Geometry check sheet. Reference: the model listing, model coordinates, mm. Face numbers are marked on the shaded views. A direction names the side the tool comes from. Coordinates: 2 decimals unless noted, no trailing zeros. Order: outer loops, then holes, each group sorted by start corner. A loop starts at its lowest first (then second) coordinate and runs counter-clockwise, first axis right, second up. Notation, with made-up numbers: (67.5, 87.25) -> (121.5, 87.25) arc R26 cw to (121.5, 110.25) -> close; hole circle Ø11 at (13, 44). An arc over 180 degrees is marked (long way). Answer in a Markdown table with one row per item. Add a question column.
```python
from build123d import *

# Parameters (mm, degrees)
F0_W      = 67.5
F0_H      = 19.4
F1_DEPTH  = 50
F3_DEPTH  = 17.5
F4_R      = 12
F5_DEPTH  = 1.9
F7_DEPTH  = 1.25
F8_DEPTH  = 11
F9_R      = 7
F11_DEPTH = 8
F12_R     = 5
F14_DEPTH = 1.25


with BuildPart() as f1:
    # F0 (on Top) → F1 (new body)
    with BuildSketch(Plane.XY):
        Rectangle(F0_W, F0_H)
    extrude(amount=F1_DEPTH)

    # F2 (on face) → F3 (cut)
    with BuildSketch(Plane.XZ.offset(9.7)):
        with BuildLine():
            Line((-6.1, 31.5), (-6.1, 30.5))
            Line((-6.1, 30.5), (-29.5, 30.5))
            ThreePointArc((-29.5, 30.5), (-31.62132, 29.62132), (-32.5, 27.5))
            Line((-32.5, 27.5), (-32.5, 1.5))
            Line((-32.5, 1.5), (0, 1.5))
            Line((0, 1.5), (32.5, 1.5))
            Line((32.5, 1.5), (32.5, 27.5))
            ThreePointArc((32.5, 27.5), (31.62132, 29.62132), (29.5, 30.5))
            Line((29.5, 30.5), (6.1, 30.5))
            Line((6.1, 30.5), (6.1, 31.5))
            Line((6.1, 31.5), (5.1, 31.5))
            Line((5.1, 31.5), (0, 31.5))
            Line((0, 31.5), (-5.1, 31.5))
            Line((-5.1, 31.5), (-6.1, 31.5))
        make_face()
    extrude(amount=-F3_DEPTH, mode=Mode.SUBTRACT)

    # F4 (on face) → F5 (cut, through all)
    with BuildSketch(Plane.XZ.offset(-7.8)):
        with Locations((0, 16)):
            Circle(F4_R)
    extrude(amount=-F5_DEPTH, mode=Mode.SUBTRACT)

    # F6 (on face) → F7 (cut, through all)
    with BuildSketch(Plane(origin=(-33.75, 0, 0), x_dir=(0, -1, 0), z_dir=(-1, 0, 0))):
        with BuildLine():
            Line((3.45, 26.5), (0.95, 26.5))
            ThreePointArc((0.95, 26.5), (-1.17132, 25.62132), (-2.05, 23.5))
            Line((-2.05, 23.5), (-2.05, 12.5))
            ThreePointArc((-2.05, 12.5), (-1.17132, 10.37868), (0.95, 9.5))
            Line((0.95, 9.5), (3.45, 9.5))
            ThreePointArc((3.45, 9.5), (5.57132, 10.37868), (6.45, 12.5))
            Line((6.45, 12.5), (6.45, 23.5))
            ThreePointArc((6.45, 23.5), (5.57132, 25.62132), (3.45, 26.5))
        make_face()
    extrude(amount=-F7_DEPTH, mode=Mode.SUBTRACT)

    # F2 (on face) → F8 (cut)
    with BuildSketch(Plane.XZ.offset(9.7)):
        Polygon((-5.1, 50), (-5.1, 31.5), (0, 31.5), (5.1, 31.5), (5.1, 50), (0, 50), align=None)
    extrude(amount=-F8_DEPTH, mode=Mode.SUBTRACT)

    # F9
    f9_edges = [f1.edges().sort_by_distance(p)[0] for p in [
        (32.5, -0.95, 1.5),
        (-33.75, 0, 0),
        (-32.5, -0.95, 1.5),
        (33.75, 0, 0),
    ]]
    fillet(f9_edges, radius=F9_R)

    # F10 (on face) → F11 (join)
    with BuildSketch(Plane.XY.offset(50)):
        Polygon((10, 9.7), (0, 9.7), (-10, 9.7), (-10, 2.7), (0, 2.7), (10, 2.7), align=None)
    extrude(amount=F11_DEPTH)

    # F12
    f12_edges = [f1.edges().sort_by_distance(p)[0] for p in [
        (10, 6.2, 58),
        (-10, 6.2, 58),
    ]]
    fillet(f12_edges, radius=F12_R)

    # F13 (on face) → F14 (cut, through all)
    with BuildSketch(Plane.YZ.offset(33.75)):
        with BuildLine():
            Line((-2.2, 27), (-4.2, 27))
            ThreePointArc((-4.2, 27), (-6.32132, 26.12132), (-7.2, 24))
            Line((-7.2, 24), (-7.2, 13))
            ThreePointArc((-7.2, 13), (-6.32132, 10.87868), (-4.2, 10))
            Line((-4.2, 10), (-2.2, 10))
            ThreePointArc((-2.2, 10), (-0.07868, 10.87868), (0.8, 13))
            Line((0.8, 13), (0.8, 24))
            ThreePointArc((0.8, 24), (-0.07868, 26.12132), (-2.2, 27))
        make_face()
    extrude(amount=-F14_DEPTH, mode=Mode.SUBTRACT)


solid = f1.part
```
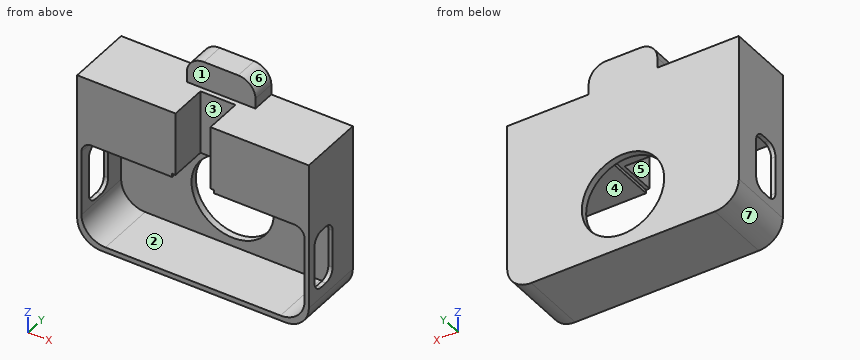
(1) Access from +Z, -Z, +X, -X, +Y, -Y to the whole of each face (thin tool, end or side, straight path). Record for the marked faces 1, 2 and 3.
(2) Mould release check, pull along Z, two halves, no side actions. Record for the marked faces 4, 5, 6 and 7: +Z half, -Z half, draft (parallel to the pull), parting line (faces both ways), or undercut.
(3) Scan lines: line 1 along Z through (x, y) = (0, 8.65); line 2 along Z through (x, y) = (-13, 0); line 3 along X through (y, z) = (-7, 37). Record each from-to range of solid material in increasing order.
(4) Cross-section at D-D (x = 15). Enter the section's corners in (y, z), plus the area to 4 significant figures.
(5) Cross-section at C-C (z = 16). Enter the section's corners in (x, y), plus the area to 3 significant figures.
(6) Go/stop test with flat-tipped pins: P1, Ø1.4, axis at x = 33.5, y = -3, coming from the -Z side; P2, Ø1.5, axis at y = 7, z = 51, coming from the -X side; P3, Ø1.4, axis at x = 33, y = -2.5, coming from the +Z side. Record where each tip stops, or that it passes through.
(7) Cross-section at B-B (y = 4.5). Enter the section's corners in (x, z), plus the area to 3 significant figures.
(8) Cross-section at A-A (x = 0). Enter the section's corners in (y, z).
Checks:
| question | item | result |
|---|---|---|
| 1 | face 1 | +Z, +X, -X, -Y |
| 1 | face 2 | -Y |
| 1 | face 3 | +Z, -Y |
| 2 | face 4 | undercut |
| 2 | face 5 | draft |
| 2 | face 6 | +Z half |
| 2 | face 7 | -Z half |
| 3 | line 1 | 0 to 4, 28 to 58 |
| 3 | line 2 | 0 to 1.5, 30.5 to 50 |
| 3 | line 3 | -33.75 to -5.1, 5.1 to 33.75 |
| 4 | outline | (-9.7, 0) -> (9.7, 0) -> (9.7, 50) -> (-9.7, 50) -> (-9.7, 30.5) -> (7.8, 30.5) -> (7.8, 1.5) -> (-9.7, 1.5) -> close |
| 4 | area | 462.5 mm² |
| 5 | outline | (-33.75, -9.7) -> (-32.5, -9.7) -> (-32.5, -6.45) -> (-33.75, -6.45) -> close; (-33.75, 2.05) -> (-32.5, 2.05) -> (-32.5, 7.8) -> (-12, 7.8) -> (-12, 9.7) -> (-33.75, 9.7) -> close; (12, 7.8) -> (32.5, 7.8) -> (32.5, 0.8) -> (33.75, 0.8) -> (33.75, 9.7) -> (12, 9.7) -> close; (32.5, -9.7) -> (33.75, -9.7) -> (33.75, -7.2) -> (32.5, -7.2) -> close |
| 5 | area | 106 mm² |
| 6 | P1 | z = 3.48 |
| 6 | P2 | x = -10 |
| 6 | P3 | z = 50 |
| 7 | outline | (-33.75, 7) arc R7 ccw to (-26.75, 0) -> (26.75, 0) arc R7 ccw to (33.75, 7) -> (33.75, 50) -> (10, 50) -> (10, 53) arc R5 ccw to (5, 58) -> (-5, 58) arc R5 ccw to (-10, 53) -> (-10, 50) -> (-33.75, 50) -> close; hole (-32.5, 8.5) arc R7 ccw to (-25.5, 1.5) -> (25.5, 1.5) arc R7 ccw to (32.5, 8.5) -> (32.5, 27.5) arc R3 ccw to (29.5, 30.5) -> (6.1, 30.5) -> (6.1, 31.5) -> (-6.1, 31.5) -> (-6.1, 30.5) -> (-29.5, 30.5) arc R3 ccw to (-32.5, 27.5) -> close |
| 7 | area | 1,630 mm² |
| 8 | outline | (-9.7, 0) -> (9.7, 0) -> (9.7, 4) -> (7.8, 4) -> (7.8, 1.5) -> (-9.7, 1.5) -> close; (1.3, 31.5) -> (7.8, 31.5) -> (7.8, 28) -> (9.7, 28) -> (9.7, 58) -> (2.7, 58) -> (2.7, 50) -> (1.3, 50) -> close |
